Build history of the part. All positions in model axes, mm. A direction names the side the tool comes from. Round coordinates to 2 decimals unless told otherwise and drop trailing zeros. Order: outer loops, then holes, each group sorted by start corner. A loop starts at its lowest first (then second) coordinate and runs counter-clockwise, first axis right, second up. Notation, with made-up numbers: (10, 39.25) -> (37, 39.25) arc R26 cw to (37, 62.25) -> close; hole circle Ø3 at (15, 75.25). An arc over 180 degrees is marked (long way). Answer as a JSON object with one key per item and string values.
from build123d import *

# Parameters (mm, degrees)
F0_W     = 76.2
F0_H     = 50.8
F1_DEPTH = 50.8
F2_W     = 0.1524
F2_H     = 12.7
F3_DEPTH = 12.7
F4_W     = 0.1524
F4_H     = 19.05
F4_H_2   = 12.7
F5_DEPTH = 50.8
F6_W     = 6.35
F6_H     = 19.05
F7_DEPTH = 3.175
F8_W     = 3.175
F8_H     = 6.35
F9_DEPTH = 25.4


with BuildPart() as f1:
    # F0 (on Front) → F1 (new body)
    with BuildSketch(Plane.XZ):
        with Locations((35.376799, 26.406373)):
            Rectangle(F0_W, F0_H)
    extrude(amount=F1_DEPTH)

    # F2 (on face) → F3 (cut)
    with BuildSketch(Plane.XZ.offset(50.8)):
        with Locations((60.700599, 45.456373)):
            Rectangle(F2_W, F2_H)
    extrude(amount=-F3_DEPTH, mode=Mode.SUBTRACT)

    # F4 (on face) → F5 (join)
    with BuildSketch(Plane.XZ.offset(38.1)):
        with Locations((60.700599, 61.331373)):
            Rectangle(F4_W, F4_H)
        with Locations((60.700599, 45.456373)):
            Rectangle(F4_W, F4_H_2)
    extrude(amount=F5_DEPTH)

    # F6 (on face) → F7 (cut)
    with BuildSketch(Plane(origin=(-2.723201, 0, 0), x_dir=(0, -1, 0), z_dir=(-1, 0, 0))):
        with Locations((3.175, 42.281373)):
            Rectangle(F6_W, F6_H)
    extrude(amount=-F7_DEPTH, mode=Mode.SUBTRACT)

    # F8 (on face) → F9 (join)
    with BuildSketch(Plane.XY.offset(32.756373)):
        Polygon((-12.248201, -6.35), (-2.723201, -6.35), (-2.723201, 0), (0.451799, 0), (0.451799, 6.35), (-12.248201, 6.35), align=None)
        with Locations((-1.135701, -3.175)):
            Rectangle(F8_W, F8_H)
    extrude(amount=F9_DEPTH)


solid = f1.part
1) Cut at D-D, the plane y = -41.5. Give the cut face in (x, z).
Checked values:
{"outline": "(-2.72, 1.01) -> (73.48, 1.01) -> (73.48, 51.81) -> (60.78, 51.81) -> (60.78, 70.86) -> (60.62, 70.86) -> (60.62, 51.81) -> (-2.72, 51.81) -> close"}
2) Which spindle directions (+Z, -Z, +X, -X, +Y, -Y) get a long thin tool onto all of the face, cutting with end or side? Do faces 1 (the face through (0.452, 3, 48)), 2 (the face through (60.777, -63, 55)), 3 (the face through (60.624, -63, 55)). Say none if no direction does.
Checked values:
{"face 1": "+Z, +X, +Y", "face 2": "+Z, +X, -Y", "face 3": "+Z, -X, -Y"}
3) Probe L1, parallel to X at y = -27, z = 28.5; L2, parallel to Y at x = 27.5, z = 31; L3, parallel to Z at x = 8, y = -16. List the from-to ranges inside material, lowest first. Write a range as from..to.
Checked values:
{"L1": "x = -2.72..73.48", "L2": "y = -50.8..0", "L3": "z = 1.01..51.81"}
4) Cut at C-C, the plane x = 59. Give the cut face in (y, z), plus the area to 3 significant figures.
Checked values:
{"outline": "(-50.8, 1.01) -> (0, 1.01) -> (0, 51.81) -> (-50.8, 51.81) -> close", "area": "2,580 mm²"}
5) Cut at B-B, the plane z = 42. Give the cut face in (x, y), plus the area to 3 significant figures.
Checked values:
{"outline": "(-12.25, -6.35) -> (-2.72, -6.35) -> (-2.72, -50.8) -> (60.62, -50.8) -> (60.62, -88.9) -> (60.78, -88.9) -> (60.78, -50.8) -> (73.48, -50.8) -> (73.48, 0) -> (0.45, 0) -> (0.45, 6.35) -> (-12.25, 6.35) -> close", "area": "4,020 mm²"}
6) Flat gauge pins, fed straight in: pin 1 Ø8 at (x, z) = (55.5, 34) entering from +Y; pin 2 Ø8 at (y, z) = (-50, 60) entering from -X; pin 3 Ø5 at (x, z) = (15.5, 40.5) entering from -Y. Where does each tip first touch, or does it go through?
Checked values:
{"pin 1": "stops at y = 0", "pin 2": "stops at x = 60.62", "pin 3": "stops at y = -50.8"}
7) Cut at A-A, the plane y = -5. Give the cut face in (x, z).
Checked values:
{"outline": "(-12.25, 32.76) -> (-2.72, 32.76) -> (-2.72, 1.01) -> (73.48, 1.01) -> (73.48, 51.81) -> (0.45, 51.81) -> (0.45, 58.16) -> (-12.25, 58.16) -> close"}
